```python
from build123d import *

# Parameters (mm, degrees)
SKETCH_2_R          = 17.9
EXTRUDE_1_DEPTH     = 50
SKETCH_3_R          = 6.5
EXTRUDE_2_DEPTH     = 4.5
SKETCH_4_R          = 1.585
EXTRUDE_5_DEPTH     = 12.5
SKETCH_5_R          = 1.5
CUT_EXTRUDE_1_DEPTH = 0.5
SKETCH_6_W          = 3.8
SKETCH_6_H          = 0.5
EXTRUDE_6_DEPTH     = 7


with BuildPart() as part:
    # ｽｹｯﾁ2 → ﾎﾞｽ - 押し出し1 (new body)
    with BuildSketch(Plane.XY):
        Circle(SKETCH_2_R)
    extrude(amount=EXTRUDE_1_DEPTH)

    # ｽｹｯﾁ3 → ﾎﾞｽ - 押し出し2 (add)
    with BuildSketch(Plane.XY.offset(50)):
        Circle(SKETCH_3_R)
    extrude(amount=EXTRUDE_2_DEPTH)

    # ｽｹｯﾁ4 → ﾎﾞｽ - 押し出し5 (add)
    with BuildSketch(Plane.XY.offset(54.5)):
        Circle(SKETCH_4_R)
    extrude(amount=EXTRUDE_5_DEPTH)

    # ｽｹｯﾁ5 → ｶｯﾄ - 押し出し1 (cut)
    with BuildSketch(Plane.XY.offset(50)):
        with Locations((0, 12.5)):
            Circle(SKETCH_5_R)
        with Locations((0, -12.5)):
            Circle(SKETCH_5_R)
    extrude(amount=-CUT_EXTRUDE_1_DEPTH, mode=Mode.SUBTRACT)

    # ｽｹｯﾁ6 → ﾎﾞｽ - 押し出し6 (add)
    with BuildSketch(Plane(origin=(0, 0, 0), x_dir=(-1, 0, 0), z_dir=(0, 0, -1))):
        with Locations((0, 13.7)):
            Rectangle(SKETCH_6_W, SKETCH_6_H)
        with Locations((0, -13.7)):
            Rectangle(SKETCH_6_W, SKETCH_6_H)
    extrude(amount=EXTRUDE_6_DEPTH)


solid = part.part
```
The model under review builds one solid part; all positions refer to its coordinate system, in mm. A direction names the side the tool comes from. Give positions to 0.01 mm unless a question says otherwise; leave off trailing zeros. Write each loop counter-clockwise with the first axis right and the second up, starting at its lowest first coordinate (ties: lowest second). Pieces come first, ordered by that corner, then holes. Notation, with made-up numbers: (74, 33.5) - (127, 33.5) arc R19 ccw to (127, 54.5) - close; hole circle Ø1 at (14.25, 37.25). An arc over 180 degrees is marked (long way). Answer in a Markdown table with one row per item. Add a question column.
1. Insertion check: P1, Ø1.8, axis at x = 0, y = -12.5, coming from the +Z side; P2, Ø1.1, axis at x = -0.5, z = -3.5, coming from the +Y side; P3, Ø8, axis at x = 4.5, z = 40.5, coming from the -Y side. Each pin has a flat end and moves straight along its axis. Give the tip position at first contact, or say it passes through.
2. We need section D-D on y = -12.5. Write out the cut boundary in (x, z), then the cut area to 3 significant figures.
3. We need section B-B on y = 0. Write out the cut boundary in (x, z) (3 decimals), then the cut area to 3 significant figures.
4. Draft analysis for pull direction X (two halves, no side actions). For faces 1 (the cylindrical face through (-5.158, -3.955, 52.218)), 2 (the cylindrical face through (-0.325, 11.036, 49.754)), 3 (the flat face through (8, 0, 50)), state which applies: +X half, -X half, draft (parallel to the pull), parting line (faces both ways), or undercut.
5. Tool access review of faces 4 (the flat face through (0, -13.45, -3)), 5 (the cylindrical face through (-14.2, -10.9, 24.6)), 6 (the flat face through (0, -13.95, -3)), 7 (the flat face through (1.4, -1.4, 54.5)), 8 (the flat face through (0, 13.95, -3)): name each direction out of +Z, -Z, +X, -X, +Y, -Y from which nothing blocks a thin tool from reaching the whole face with its end or side.
6. Wall thickness on line 1 along Y through (x, z) = (0, 49.8); line 2 along Z through (x, y) = (-8, 3); line 3 along Y through (x, z) = (0, 3): over which ranges is each line inside the solid? List them lowest first. Write a range as [from, to].
7. We need section A-A on x = 0. Write out the cut boundary in (y, z) (3 decimals).
8. We need section C-C on z = 52.5. Write out the cut boundary in (x, y).
Ans:
| question | item | result |
|---|---|---|
| 1 | P1 | stops at z = 49.5 |
| 1 | P2 | stops at y = 13.95 |
| 1 | P3 | stops at y = -17.89 |
| 2 | outline | (-12.81, 0) - (12.81, 0) - (12.81, 50) - (1.5, 50) - (1.5, 49.5) - (-1.5, 49.5) - (-1.5, 50) - (-12.81, 50) - close |
| 2 | area | 1,280 mm^2 |
| 3 | outline | (-17.9, 0) - (17.9, 0) - (17.9, 50) - (6.5, 50) - (6.5, 54.5) - (1.585, 54.5) - (1.585, 67) - (-1.585, 67) - (-1.585, 54.5) - (-6.5, 54.5) - (-6.5, 50) - (-17.9, 50) - close |
| 3 | area | 1,890 mm^2 |
| 4 | face 1 | parting line |
| 4 | face 2 | undercut |
| 4 | face 3 | draft |
| 5 | face 4 | -Z, +X, -X |
| 5 | face 5 | +Z, -Z |
| 5 | face 6 | -Z, +X, -X, -Y |
| 5 | face 7 | +Z |
| 5 | face 8 | -Z, +X, -X, +Y |
| 6 | line 1 | y = [-17.9, -14], [-11, 11], [14, 17.9] |
| 6 | line 2 | z = [0, 50] |
| 6 | line 3 | y = [-17.9, 17.9] |
| 7 | outline | (-17.9, 0) - (-13.95, 0) - (-13.95, -7) - (-13.45, -7) - (-13.45, 0) - (13.45, 0) - (13.45, -7) - (13.95, -7) - (13.95, 0) - (17.9, 0) - (17.9, 50) - (14, 50) - (14, 49.5) - (11, 49.5) - (11, 50) - (6.5, 50) - (6.5, 54.5) - (1.585, 54.5) - (1.585, 67) - (-1.585, 67) - (-1.585, 54.5) - (-6.5, 54.5) - (-6.5, 50) - (-11, 50) - (-11, 49.5) - (-14, 49.5) - (-14, 50) - (-17.9, 50) - close |
| 8 | outline | circle Ø13 at (0, 0) |
